Read the model definition and answer for the solid it produces. Units are mm, in the model's axes. Face numbers are marked on the shaded views. A direction names the side the tool comes from. Coordinates: 2 decimals unless noted, no trailing zeros. Order: outer loops, then holes, each group sorted by start corner. A loop starts at its lowest first (then second) coordinate and runs counter-clockwise, first axis right, second up. Notation, with made-up numbers: M 61,-8.5 L 72,-8.5 A19 ccw 72,17.5 Z; hole C 31,-21 d9. An arc over 180 degrees is marked long. Write each question's results on one line, items separated by ' | '.
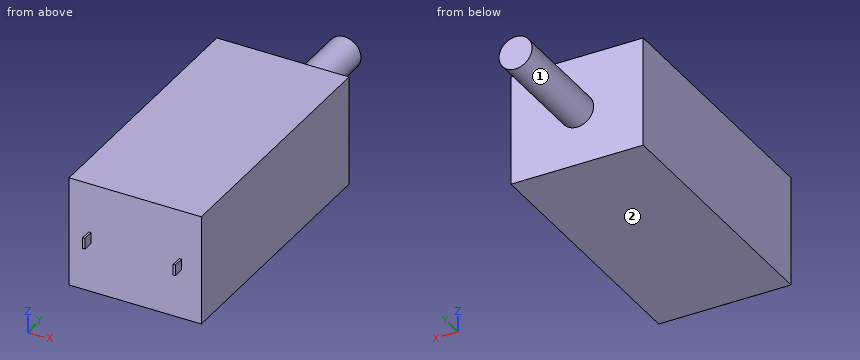
```python
from build123d import *

# Parameters (mm, degrees)
SKETCH1_W           = 24
SKETCH1_H           = 12
BOSS_EXTRUDE1_DEPTH = 5
SKETCH2_R           = 1.5
BOSS_EXTRUDE2_DEPTH = 10
SKETCH3_W           = 0.2
SKETCH3_H           = 1
BOSS_EXTRUDE3_DEPTH = 1


with BuildPart() as part:
    # Sketch1 → Boss-Extrude1 (new, symmetric)
    with BuildSketch(Plane(origin=(0, 0, 0), x_dir=(0, 1, 0), z_dir=(0, 0, 1))):
        Rectangle(SKETCH1_W, SKETCH1_H)
    extrude(amount=BOSS_EXTRUDE1_DEPTH, both=True)

    # Sketch2 → Boss-Extrude2 (add)
    with BuildSketch(Plane(origin=(0, 12, 0), x_dir=(-1, 0, 0), z_dir=(0, 1, 0))):
        with Locations(Location((0, 0, 0), (0, 0, 90))):
            Circle(SKETCH2_R)
    extrude(amount=BOSS_EXTRUDE2_DEPTH)

    # Sketch3 → Boss-Extrude3 (add)
    with BuildSketch(Plane.XZ.offset(12)):
        with Locations((4.1, 0)):
            Rectangle(SKETCH3_W, SKETCH3_H)
        with Locations((-4.1, 0)):
            Rectangle(SKETCH3_W, SKETCH3_H)
    extrude(amount=BOSS_EXTRUDE3_DEPTH)


solid = part.part
```
(1) The part is cut by section B-B, the plane z = 0. Write down the section's boundary in (x, y), then the cut area to 3 significant figures.
Conclusion:
outline: M -6,-12 L -4.2,-12 L -4.2,-13 L -4,-13 L -4,-12 L 4,-12 L 4,-13 L 4.2,-13 L 4.2,-12 L 6,-12 L 6,12 L 1.5,12 L 1.5,22 L -1.5,22 L -1.5,12 L -6,12 Z | area: 318 mm²
(2) The part is cut by section A-A, the plane x = 0. Write down the section's boundary in (y, z), then the cut area to 3 significant figures.
Conclusion:
outline: M -12,-5 L 12,-5 L 12,-1.5 L 22,-1.5 L 22,1.5 L 12,1.5 L 12,5 L -12,5 Z | area: 270 mm²
(3) The part is cut by section D-D, the plane x = -3. Write down the section's boundary in (y, z), then the cut area to 3 significant figures.
Conclusion:
outline: M -12,-5 L 12,-5 L 12,5 L -12,5 Z | area: 240 mm²
(4) For the marked faces 1 and 2, determine the directions among +Z, -Z, +X, -X, +Y, -Y from which every point of the face is accessible in a straight line to the end or side of a thin tool.
Conclusion:
face 1: +Y | face 2: -Z, +X, -X, +Y, -Y
(5) Straight lines are drawn through the part: line 1 (Y direction, x = 0.5, z = 3.5); line 2 (Z direction, x = -1.25, y = 12.5). For each, find the intervals that lie inside material, in ascending order.
Conclusion:
line 1: -12 to 12 | line 2: -0.83 to 0.83
(6) The part is cut by section C-C, the plane y = 16. Write down the section's boundary in (x, z), then the cut area to 3 significant figures.
Conclusion:
outline: C 0,0 d3 | area: 7.07 mm²
(7) Given pin 1 (1.5 mm diameter, centred on x = 4, z = 3.5, fed in from +Y); pin 2 (6 mm diameter, centred on x = -0.5, z = -3.5, fed in from -Y); pin 3 (0.5 mm diameter, centred on y = -12.5, z = 0, fed in from -X), each flat-ended and moving along its own axis, determine where each tip first touches the part or whether it passes through.
Conclusion:
pin 1: y = 12 | pin 2: y = -12 | pin 3: x = -4.2
